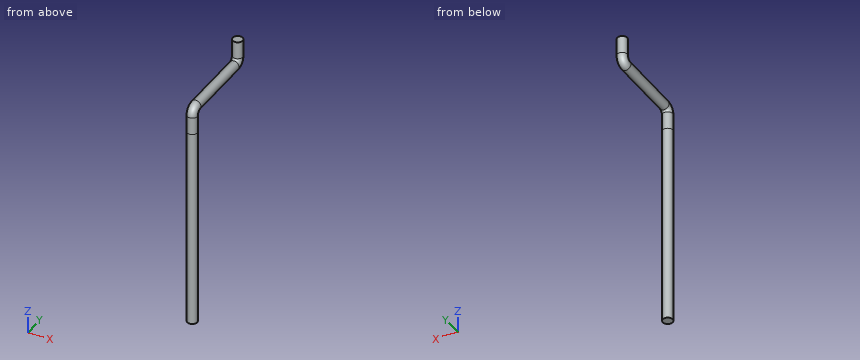
```python
from build123d import *

# Parameters (mm, degrees)
CROQUIS1_R              = 7.5
CROQUIS2_R              = 7.5
SALIENTE_EXTRUIR1_DEPTH = 300


with BuildPart() as part:
    # Barrer1: sweep along a curve in space
    with BuildLine() as barrer1_path:
        Line((4.693833182, 15.151479833, 0), (4.693833182, 15.151479833, 26))
        ThreePointArc((4.693833182, 15.151479833, 26), (4.693833182, 18.080412022, 33.071067812), (4.693833182, 25.151479833, 36))
        Line((4.693833182, 25.151479833, 36), (4.693833182, 130.151479833, 36))
        ThreePointArc((4.693833182, 130.151479833, 36), (4.693833182, 137.222547645, 38.928932188), (4.693833182, 140.151479833, 46))
        Line((4.693833182, 140.151479833, 46), (4.693833182, 140.151479833, 72))
    # Croquis1 → Barrer1 (sweep)
    with BuildSketch(Plane.XY):
        with Locations((4.693833182, 15.151479833)):
            Circle(CROQUIS1_R)
    sweep(path=barrer1_path.line)

    # Croquis2 → Saliente-Extruir1 (add)
    with BuildSketch(Plane(origin=(0, 0, 0), x_dir=(-1, 0, 0), z_dir=(0, 0, -1))):
        with Locations((-4.693833182, 15.151479833)):
            Circle(CROQUIS2_R)
    extrude(amount=SALIENTE_EXTRUIR1_DEPTH)


solid = part.part
```
Part model, mm, in its own coordinate system. Round coordinates to 2 decimals unless told otherwise and drop trailing zeros. Loops run counter-clockwise (first coordinate to the right, second up) from the corner with the lowest first, then second, coordinate; pieces in that order, holes last.
Item 1: Drop flat-ended pins along their axis: P1, Ø6, axis at x = 4.5, z = 25, coming from the +Y side; P2, Ø3, axis at x = 1, y = 121.5, coming from the -Z side; P3, Ø4, axis at x = 8.5, z = 12, coming from the -Y side. Give the stop position or say it passes through.
Item 2: Drill centre lines: line 1 (Y direction, x = 4.75, z = -85); line 2 (Z direction, x = 4, y = 115); line 3 (Y direction, x = 6.5, z = -8). Where is each one in solid material? Low to high.
Item 3: Cut at A-A, the plane x = 5.25. Give the cut face in (y, z), then the cut area to 3 significant figures.
Item 4: Cut at C-C, the plane z = 10.5. Give the cut face in (x, y).
Item 5: Cut at B-B, the plane y = 116. Give the cut face in (x, z), then the cut area to 3 significant figures.
A:
1. P1: stops at y = 23.65
1. P2: stops at z = 28.83
1. P3: stops at y = 7.87
2. line 1: y = 7.65 to 22.65
2. line 2: z = 28.53 to 43.47
2. line 3: y = 7.87 to 22.43
3. outline: (7.67, -300) - (22.63, -300) - (22.63, 26) arc R2.52 cw to (25.15, 28.52) - (130.15, 28.52) arc R17.48 ccw to (147.63, 46) - (147.63, 72) - (132.67, 72) - (132.67, 46) arc R2.52 cw to (130.15, 43.48) - (25.15, 43.48) arc R17.48 ccw to (7.67, 26) - close
3. area: 7,310 mm2
4. outline: circle Ø15 at (4.69, 15.15)
5. outline: circle Ø15 at (4.69, 36)
5. area: 177 mm2
